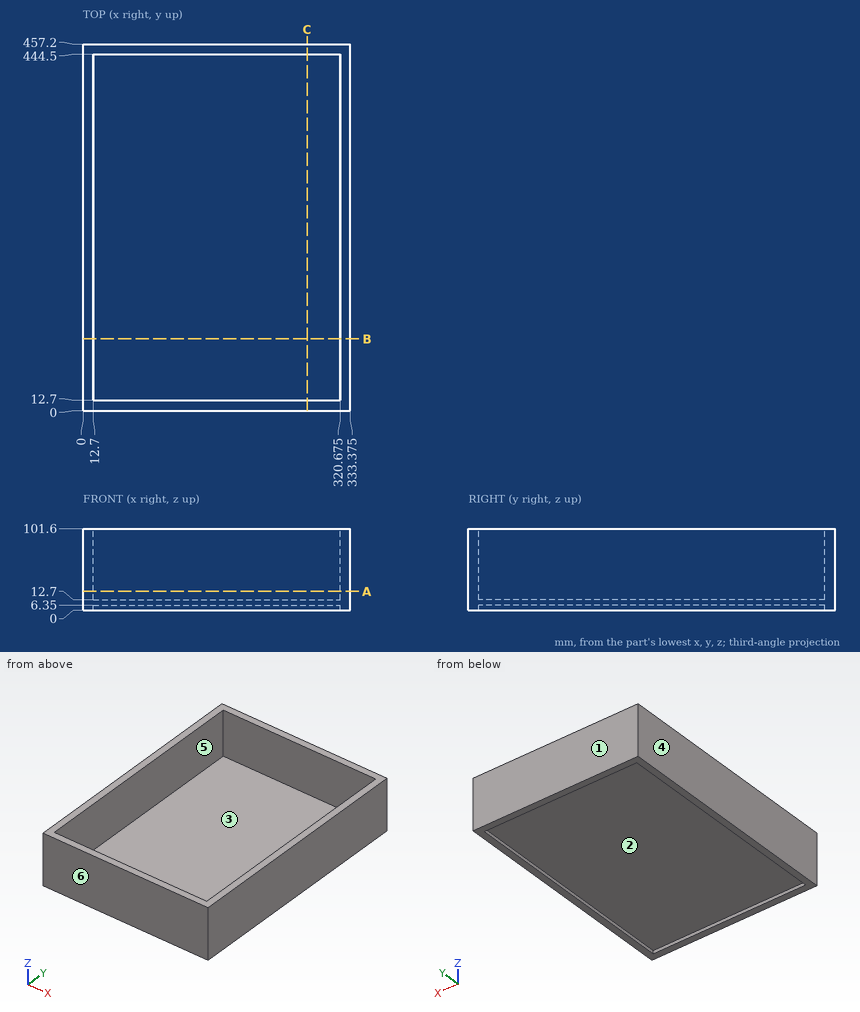
The drawing under review shows one solid part. Ordinate dimensions are in mm from its lowest x, y, z. A direction names the side the tool comes from. Coordinates: 2 decimals unless noted, no trailing zeros. Order: outer loops, then holes, each group sorted by start corner. A loop starts at its lowest first (then second) coordinate and runs counter-clockwise, first axis right, second up. Notation, with made-up numbers: (17.25, 53) -> (69.25, 53) arc R15 ccw to (69.25, 63) -> close; hole circle Ø1 at (54, 77.25). An arc over 180 degrees is marked (long way). Answer as CSV lines item,"result".
Q1. We need section C-C (x = 279.5). State the section outline as (y, z) points.
Model answer:
outline,"(0, 0) -> (12.7, 0) -> (12.7, 6.35) -> (444.5, 6.35) -> (444.5, 0) -> (457.2, 0) -> (457.2, 101.6) -> (444.5, 101.6) -> (444.5, 12.7) -> (12.7, 12.7) -> (12.7, 101.6) -> (0, 101.6) -> close"
Q2. Clearance check with flat-ended pins moving along their axes: pin 1 Ø8 at (x, y) = (142.5, 52.5) entering from +Z; pin 2 Ø2 at (x, y) = (235.5, 286.5) entering from -Z. State where each tip first meets the part, or that it passes through.
Model answer:
pin 1,"stops at z = 12.7"
pin 2,"stops at z = 6.35"
Q3. For the marked faces 5 and 6, list the 3-axis set-ups (+Z, -Z, +X, -X, +Y, -Y) from which the entire face can be reached by the end or side of a thin tool; tool diameter is ignored.
Model answer:
face 5,"+Z"
face 6,"+Z, -Z, +X, -X, -Y"
Q4. We need section A-A (z = 23.5). State the section outline as (x, y) points (3 decimals).
Model answer:
outline,"(0, 0) -> (333.375, 0) -> (333.375, 457.2) -> (0, 457.2) -> close; hole (12.7, 12.7) -> (320.675, 12.7) -> (320.675, 444.5) -> (12.7, 444.5) -> close"
Q5. Wall thickness on line 1 along X through (y, z) = (115.5, 26.5) (3 decimals); line 2 along Y through (x, z) = (296, 86); line 3 along Z through (x, y) = (50.5, 39.5): over which ranges is each line inside the solid? List them lowest first. Write a range as [from, to].
Model answer:
line 1,"x = [0, 12.7], [320.675, 333.375]"
line 2,"y = [0, 12.7], [444.5, 457.2]"
line 3,"z = [6.35, 12.7]"
Q6. Draft analysis for pull direction X (two halves, no side actions). For the marked faces 1, 2, 3 and 4, state which applies: released by +X, released by -X, zero draft, split by the parting line, or undercut.
Model answer:
face 1,"zero draft"
face 2,"undercut"
face 3,"undercut"
face 4,"released by -X"
Q7. We need section B-B (y = 89.5). State the section outline as (x, z) points (3 decimals).
Model answer:
outline,"(0, 0) -> (12.7, 0) -> (12.7, 6.35) -> (320.675, 6.35) -> (320.675, 0) -> (333.375, 0) -> (333.375, 101.6) -> (320.675, 101.6) -> (320.675, 12.7) -> (12.7, 12.7) -> (12.7, 101.6) -> (0, 101.6) -> close"
